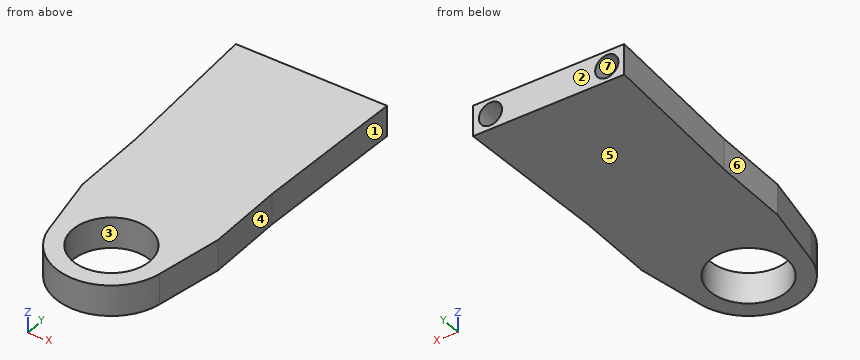
```python
from build123d import *

# Parameters (mm, degrees)
SKETCH1_R           = 5
BOSS_EXTRUDE1_DEPTH = 2
SKETCH2_W           = 17.5
SKETCH2_H           = 4
BOSS_EXTRUDE2_DEPTH = 30
BOSS_EXTRUDE3_DEPTH = 2
SKETCH3_R           = 1.5
CUT_EXTRUDE1_DEPTH  = 6


with BuildPart() as part:
    # Sketch1 → Boss-Extrude1 (new, symmetric)
    with BuildSketch(Plane.XY):
        with BuildLine():
            Line((8.75, 7.25), (-8.75, 7.25))
            Line((-8.75, 7.25), (-7.123668925, -1.347531462))
            ThreePointArc((-7.123668925, -1.347531462), (0, -7.25), (7.123668925, -1.347531462))
            Line((7.123668925, -1.347531462), (8.75, 7.25))
        make_face()
        Circle(SKETCH1_R, mode=Mode.SUBTRACT)
    extrude(amount=BOSS_EXTRUDE1_DEPTH, both=True)

    # Sketch2 → Boss-Extrude2 (add)
    with BuildSketch(Plane(origin=(0, 7.25, 0), x_dir=(1, 0, 0), z_dir=(0, 1, 0))):
        Rectangle(SKETCH2_W, SKETCH2_H)
    extrude(amount=BOSS_EXTRUDE2_DEPTH)

    # Sketch4 → Boss-Extrude3 (add, symmetric)
    with BuildSketch(Plane.XY):
        Polygon((-8.75, 37.25), (-9.75, 37.25), (-8.75, 17.25), align=None)
        Polygon((8.75, 37.25), (9.75, 37.25), (8.75, 17.25), align=None)
    extrude(amount=BOSS_EXTRUDE3_DEPTH, both=True)

    # Sketch3 → Cut-Extrude1 (cut)
    with BuildSketch(Plane(origin=(0, 37.25, 0), x_dir=(1, 0, 0), z_dir=(0, 1, 0))):
        with Locations(Location((-7.5, 0, 0), (0, 0, 180))):
            Circle(SKETCH3_R)
        with Locations(Location((7.5, 0, 0), (0, 0, 180))):
            Circle(SKETCH3_R)
    extrude(amount=-CUT_EXTRUDE1_DEPTH, mode=Mode.SUBTRACT)


solid = part.part
```
Build history of the part. All positions in model axes, mm. Face numbers are marked on the shaded views. A direction names the side the tool comes from. Give positions to 0.01 mm unless a question says otherwise; leave off trailing zeros. Order: outer loops, then holes, each group sorted by start corner. A loop starts at its lowest first (then second) coordinate and runs counter-clockwise, first axis right, second up. Notation, with made-up numbers: M 33.25,-9.5 L 65.25,-9.5 A23 ccw 65.25,13.5 Z; hole C 26,8.25 d2. An arc over 180 degrees is marked long. Return JSON: item names as keys, results as strings.
Q1. Band-saw the part on B-B (z = 0). Give the cut face in (x, y).
Answer list:
{"outline": "M -9.75,37.25 L -8.75,17.25 L -8.75,7.25 L -7.12,-1.35 A7.25 ccw 7.12,-1.35 L 8.75,7.25 L 8.75,17.25 L 9.75,37.25 L 9,37.25 L 9,31.25 L 6,31.25 L 6,37.25 L -6,37.25 L -6,31.25 L -9,31.25 L -9,37.25 Z; hole C 0,0 d10"}
Q2. Band-saw the part on D-D (y = 32). Give the cut face in (x, z), then the cut area to 3 significant figures.
Answer list:
{"outline": "M -9.49,-2 L 9.49,-2 L 9.49,2 L -9.49,2 Z; hole C -7.5,0 d3; hole C 7.5,0 d3", "area": "61.8 mm^2"}
Q3. Flat gauge pins, fed straight in: pin 1 (9 mm diameter, centred on x = 0, y = 0, fed in from +Z); pin 2 (2 mm diameter, centred on x = 5.5, z = 0, fed in from -Y); pin 3 (1 mm diameter, centred on y = 29.5, z = 1, fed in from -X); pin 4 (2 mm diameter, centred on y = 14.5, z = -1, fed in from -X). Where does each tip first touch, or does it go through?
Answer list:
{"pin 1": "passes through", "pin 2": "stops at y = -5.68", "pin 3": "stops at x = -9.39", "pin 4": "stops at x = -8.75"}
Q4. 3-axis set-ups, long thin cutter, end or side, ignore diameter. For the marked faces 4, 5, 6 and 7: which of +Z, -Z, +X, -X, +Y, -Y reach the whole face in a straight line?
Answer list:
{"face 4": "+Z, -Z, +X, -Y", "face 5": "-Z, +X, -X, +Y, -Y", "face 6": "+Z, -Z, -X, -Y", "face 7": "+Y"}
Q5. Band-saw the part on A-A (x = 0). Give the cut face in (y, z), then the cut area to 3 significant figures.
Answer list:
{"outline": "M -7.25,-2 L -5,-2 L -5,2 L -7.25,2 Z; M 5,-2 L 37.25,-2 L 37.25,2 L 5,2 Z", "area": "138 mm^2"}
Q6. Two-plate mould, pull along X, no slides. Class the marked faces 1, 2 and 3: pulls with the +X half, pulls with the -X half, needs draft (parallel to the pull), parting line crosses it, or undercut.
Answer list:
{"face 1": "pulls with the +X half", "face 2": "needs draft", "face 3": "undercut"}
Q7. Band-saw the part on C-C (y = 1). Give the cut face in (x, z).
Answer list:
{"outline": "M -7.57,-2 L -4.9,-2 L -4.9,2 L -7.57,2 Z; M 4.9,-2 L 7.57,-2 L 7.57,2 L 4.9,2 Z"}
Q8. Wall check: probe 1 along Y at (x, z) = (0, -1); probe 2 along Z at (x, y) = (-7.5, 33); probe 3 along X at (y, z) = (12, -1.55). Give the ranges that are in metal, low to high. Write a range as from..to.
Answer list:
{"probe 1": "y = -7.25..-5, 5..37.25", "probe 2": "z = -2..-1.5, 1.5..2", "probe 3": "x = -8.75..8.75"}
